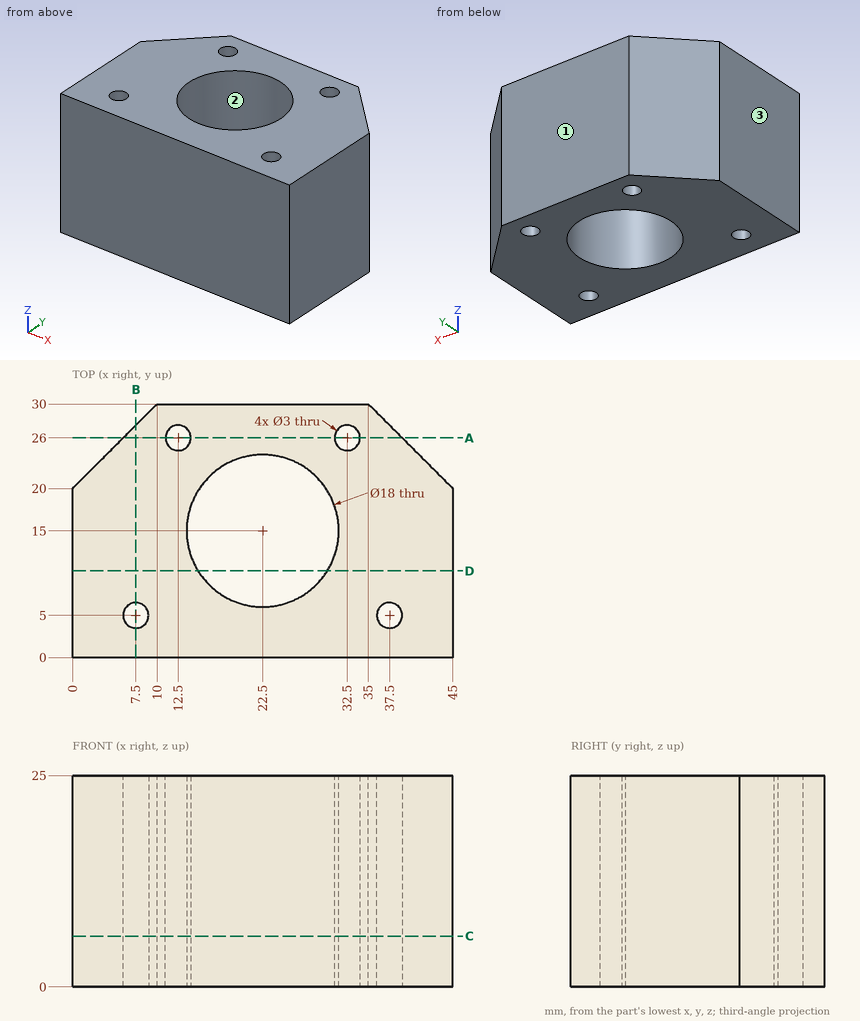
Drawing for the job (mm, zero at the part's lowest x, y, z). Give positions to 0.01 mm unless a question says otherwise; leave off trailing zeros. Loops run counter-clockwise (first coordinate to the right, second up) from the corner with the lowest first, then second, coordinate; pieces in that order, holes last. Notation, with made-up numbers: (73.25, 68.5) - (102.25, 68.5) arc R24 cw to (102.25, 97.5) - close; hole circle Ø6 at (83.5, 49). An arc over 180 degrees is marked (long way). Write item = value, one per line. Start each with the question number.
1) Probe probe 1 along Y at (x, z) = (37.5, 15); probe 2 along X at (y, z) = (5.75, 13.5); probe 3 along Y at (x, z) = (12.5, 10). List the from-to ranges inside material, lowest first. Write a range as from..to.
2) Band-saw the part on A-A on y = 26. Give the cut face in (x, z).
3) Drop flat-ended pins along their axis: pin 1 Ø6 at (y, z) = (26, 12.5) entering from +X; pin 2 Ø2.5 at (x, y) = (37.5, 5) entering from +Z. Give the stop position or say it passes through.
4) Band-saw the part on B-B on x = 7.5. Give the cut face in (y, z).
5) Pull direction X, two halves, no side cores. Call the marked faces 1, 2 and 3: +X half, -X half, draft (parallel to the pull), parting line (faces both ways), or undercut.
6) Band-saw the part on D-D on y = 10.25. Give the cut face in (x, z), plus the area to 3 significant figures.
7) Band-saw the part on C-C on z = 6. Give the cut face in (x, y), plus the area to 3 significant figures.
Final values:
q1.probe_1 = 0..3.5, 6.5..27.5
q1.probe_2 = 0..6.2, 8.8..36.2, 38.8..45
q1.probe_3 = 0..24.5, 27.5..30
q2.outline = (6, 0) - (11, 0) - (11, 25) - (6, 25) - close; (14, 0) - (31, 0) - (31, 25) - (14, 25) - close; (34, 0) - (39, 0) - (39, 25) - (34, 25) - close
q3.pin_1 = 42
q3.pin_2 = through
q4.outline = (0, 0) - (3.5, 0) - (3.5, 25) - (0, 25) - close; (6.5, 0) - (27.5, 0) - (27.5, 25) - (6.5, 25) - close
q5.face_1 = draft
q5.face_2 = undercut
q5.face_3 = -X half
q6.outline = (0, 0) - (14.86, 0) - (14.86, 25) - (0, 25) - close; (30.14, 0) - (45, 0) - (45, 25) - (30.14, 25) - close
q6.area = 743 mm²
q7.outline = (0, 0) - (45, 0) - (45, 20) - (35, 30) - (10, 30) - (0, 20) - close; hole circle Ø3 at (7.5, 5); hole circle Ø3 at (12.5, 26); hole circle Ø18 at (22.5, 15); hole circle Ø3 at (32.5, 26); hole circle Ø3 at (37.5, 5)
q7.area = 967 mm²
